Here's how the part is built. I have some questions about the finished solid (model axes, mm). Face numbers are marked on the shaded views. A direction names the side the tool comes from. Give positions to 0.01 mm unless a question says otherwise; leave off trailing zeros. Order: outer loops, then holes, each group sorted by start corner. A loop starts at its lowest first (then second) coordinate and runs counter-clockwise, first axis right, second up.
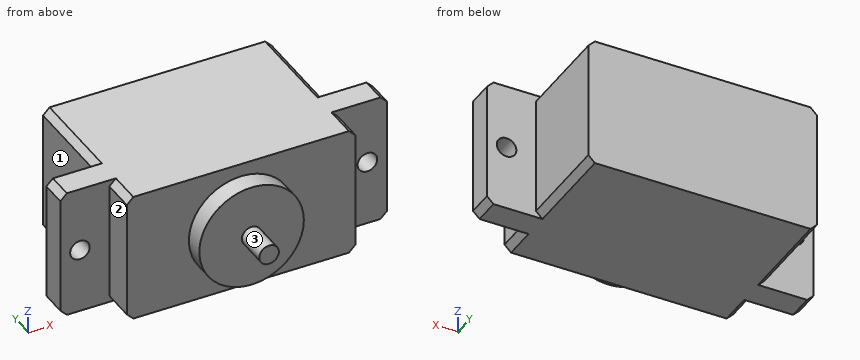
from build123d import *

# Parameters (mm, degrees)
F1_DEPTH = 40
F2_SIZE  = 2
F3_R     = 16
F4_DEPTH = 6
F5_R     = 3
F6_DEPTH = 10
F7_R     = 3
F8_DEPTH = 25


with BuildPart() as f1:
    # F0 (on Top) → F1 (new body)
    with BuildSketch(Plane.XY):
        Polygon((-50, 0), (-50, -8), (-35, -8), (-35, -18), (0, -18), (35, -18), (35, -8), (50, -8), (50, 0), (35, 0), (35, 30), (0, 30), (-35, 30), (-35, 0), align=None)
    extrude(amount=F1_DEPTH)

    # F2
    f2_edges = [f1.edges().sort_by_distance(p)[0] for p in [
        (35, 15, 40),
        (35, -13, 40),
        (50, -4, 40),
        (35, -13, 0),
        (50, -4, 0),
        (35, 15, 0),
        (-35, 15, 40),
        (-35, -13, 40),
        (-50, -4, 40),
        (-35, 15, 0),
        (-50, -4, 0),
        (-35, -13, 0),
    ]]
    chamfer(f2_edges, length=F2_SIZE)

    # F3 (on face) → F4 (join)
    with BuildSketch(Plane.XZ.offset(18)):
        with Locations((0, 20)):
            Circle(F3_R)
    extrude(amount=F4_DEPTH)

    # F5 (on face) → F6 (join)
    with BuildSketch(Plane.XZ.offset(24)):
        with Locations((0, 20)):
            Circle(F5_R)
    extrude(amount=F6_DEPTH)

    # F7 (on face) → F8 (cut)
    with BuildSketch(Plane.XZ.offset(8)):
        with Locations((-44, 20)):
            Circle(F7_R)
        with Locations((44, 20)):
            Circle(F7_R)
    extrude(amount=-F8_DEPTH, mode=Mode.SUBTRACT)


solid = f1.part
Q1. If we section it at B-B on x = 44: List the corners of the cut face in (y, z) for me, plus the area to 3 significant figures.
Filled sheet:
outline: (-8, 0) - (0, 0) - (0, 17) - (-8, 17) - close; (-8, 23) - (0, 23) - (0, 40) - (-8, 40) - close
area: 272 mm2
Q2. I need wall thicknesses on L1, parallel to Z at x = 44, y = -5.5; L2, parallel to X at y = 10.5, z = 3; L3, parallel to Y at x = -30, z = 17. Which ranges of each line are inside material? Lowest first, please.
Filled sheet:
L1: z = 0 to 17, 23 to 40
L2: x = -35 to 35
L3: y = -18 to 30
Q3. If we section it at C-C on y = -6: List the corners of the cut face in (x, z) for me.
Filled sheet:
outline: (-50, 2) - (-48, 0) - (48, 0) - (50, 2) - (50, 38) - (48, 40) - (-48, 40) - (-50, 38) - close; hole circle Ø6 at (-44, 20); hole circle Ø6 at (44, 20)
Q4. I'm going to push flat-ended pins straight in: P1, Ø13.5, axis at x = -38.5, z = 29.5, coming from the -Y side; P2, Ø9.5, axis at x = 44, z = 20, coming from the -Y side; P3, Ø2, axis at y = -24.5, z = 9, coming from the -X side. Where does each tip first touch, or does it pass through?
Filled sheet:
P1: stops at y = -18
P2: stops at y = -8
P3: stops at x = -12.38
Q5. For the marked faces 1, 2 and 3, which set-ups out of +Z, -Z, +X, -X, +Y, -Y let a thin tool reach every point of the face, with its end or its side?
Filled sheet:
face 1: +Z, -Z, -X, +Y
face 2: +Z, -Z, -X, -Y
face 3: -Y
Q6. If we section it at D-D on x = 0: List the corners of the cut face in (y, z) for me, plus the area to 3 significant figures.
Filled sheet:
outline: (-34, 17) - (-24, 17) - (-24, 4) - (-18, 4) - (-18, 0) - (30, 0) - (30, 40) - (-18, 40) - (-18, 36) - (-24, 36) - (-24, 23) - (-34, 23) - close
area: 2,170 mm2
Q7. If we section it at A-A on z = 20: List the corners of the cut face in (x, y) for me.
Filled sheet:
outline: (-50, -8) - (-47, -8) - (-47, 0) - (-50, 0) - close; (-41, -8) - (-35, -8) - (-35, -18) - (-16, -18) - (-16, -24) - (-3, -24) - (-3, -34) - (3, -34) - (3, -24) - (16, -24) - (16, -18) - (35, -18) - (35, -8) - (41, -8) - (41, 0) - (35, 0) - (35, 30) - (-35, 30) - (-35, 0) - (-41, 0) - close; (47, -8) - (50, -8) - (50, 0) - (47, 0) - close
